from build123d import *

# Parameters (mm, degrees)
BOSS_EXTRUDE7_DEPTH = 15
BOSS_EXTRUDE8_DEPTH = 5
SKETCH3_W           = 4.7625
SKETCH3_H           = 3
SKETCH3_W_2         = 3
SKETCH3_H_2         = 7.9375
CUT_EXTRUDE1_DEPTH  = 15


with BuildPart() as part:
    # Sketch1 → Boss-Extrude7 (new body)
    with BuildSketch(Plane(origin=(0, 0, 0), x_dir=(1, 0, 0), z_dir=(0, 1, 0))):
        Polygon((24.7625, 10.9375), (7.7625, 10.9375), (7.7625, 27.9375), (7.7625, 30.9375), (-3, 30.9375), (-3, 27.9375), (-3, -3), (24.7625, -3), (27.7625, -3), (27.7625, 10.9375), align=None)
        Polygon((0, 0), (4.7625, 0), (24.7625, 0), (24.7625, 7.9375), (4.7625, 7.9375), (4.7625, 27.9375), (0, 27.9375), align=None, mode=Mode.SUBTRACT)
    extrude(amount=BOSS_EXTRUDE7_DEPTH)

    # Sketch2 → Boss-Extrude8 (add)
    with BuildSketch(Plane.XZ):
        Polygon((27.7625, 3), (27.7625, -10.9375), (7.7625, -10.9375), (7.7625, -30.9375), (-3, -30.9375), (-3, 3), align=None)
    extrude(amount=BOSS_EXTRUDE8_DEPTH)

    # Sketch3 → Cut-Extrude1 (cut)
    with BuildSketch(Plane(origin=(0, 15, 0), x_dir=(1, 0, 0), z_dir=(0, 1, 0))):
        with Locations((2.38125, 29.4375)):
            Rectangle(SKETCH3_W, SKETCH3_H)
        with Locations((26.2625, 3.96875)):
            Rectangle(SKETCH3_W_2, SKETCH3_H_2)
    extrude(amount=-CUT_EXTRUDE1_DEPTH, mode=Mode.SUBTRACT)


solid = part.part
The model under review builds one solid part; all positions refer to its coordinate system, in mm. A direction names the side the tool comes from. Round coordinates to 2 decimals unless told otherwise and drop trailing zeros. Write each loop counter-clockwise with the first axis right and the second up, starting at its lowest first coordinate (ties: lowest second). Pieces come first, ordered by that corner, then holes. Notation, with made-up numbers: M 48,32.5 L 104,32.5 A16 cw 104,48.5 Z; hole C 36.25,-13.75 d1. An arc over 180 degrees is marked long. Use a Markdown table: item, result. Add a question column.
Q1. We need section A-A, the plane y = 12. State the section outline as (x, z) points.
Q2. The part is to be moulded in two halves that separate along X. For faces 4 (the face through (4.762, 7, -19)), 5 (the face through (7.762, 5, -21)), 6 (the face through (4, 0, -9)), 7 (the face through (16, 8, -7.938)), say which applies: pulls with the +X half, pulls with the -X half, needs draft (parallel to the pull), parting line crosses it, or undercut.
Q3. We need section C-C, the plane z = -16. State the section outline as (x, y) points.
Q4. Insertion check: pin 1 (4 mm diameter, centred on x = 19, y = 5.5, fed in from -Z); pin 2 (6 mm diameter, centred on y = 9.5, z = -19.5, fed in from +X). Each pin has a flat end and moves straight along its axis. Give the tip position at first contact, or say it passes through.
Q5. We need section D-D, the plane x = 2.5. State the section outline as (y, z) points, plus the area to 3 significant figures.
Q6. Machinability: for faces 1 (the face through (18, 5, -10.938)), 2 (the face through (14, 8, 0)), 3 (the face through (0, 8, -15)), which of the approach directions +Z, -Z, +X, -X, +Y, -Y give a long, thin tool a straight path to every point of the face, cutting with its end or side? Answer none if there is none.
Q7. To check wall thickness, follow line 1 (X direction, y = 9.75, z = -26); line 2 (Z direction, x = 19.5, y = 10); line 3 (Z direction, x = 5.5, y = 10.75). State the ranges of each line that lie inside material, in increasing order.
Q8. We need section B-B, the plane x = 14. State the section outline as (y, z) points, plus the area to 3 significant figures.
Findings below:
| question | item | result |
|---|---|---|
| 1 | outline | M -3,-30.94 L 0,-30.94 L 0,0 L 27.76,0 L 27.76,3 L -3,3 Z; M 4.76,-30.94 L 7.76,-30.94 L 7.76,-10.94 L 27.76,-10.94 L 27.76,-7.94 L 4.76,-7.94 Z |
| 2 | face 4 | undercut |
| 2 | face 5 | pulls with the +X half |
| 2 | face 6 | undercut |
| 2 | face 7 | needs draft |
| 3 | outline | M -3,-5 L 7.76,-5 L 7.76,15 L 4.76,15 L 4.76,0 L 0,0 L 0,15 L -3,15 Z |
| 4 | pin 1 | stops at z = -10.94 |
| 4 | pin 2 | stops at x = 7.76 |
| 5 | outline | M -5,-30.94 L 0,-30.94 L 0,0 L 15,0 L 15,3 L -5,3 Z |
| 5 | area | 215 mm² |
| 6 | face 1 | -Z, +X, +Y, -Y |
| 6 | face 2 | +X, +Y |
| 6 | face 3 | -Z, +Y |
| 7 | line 1 | x = -3 to 0, 4.76 to 7.76 |
| 7 | line 2 | z = -10.94 to -7.94, 0 to 3 |
| 7 | line 3 | z = -30.94 to -7.94, 0 to 3 |
| 8 | outline | M -5,-10.94 L 15,-10.94 L 15,-7.94 L 0,-7.94 L 0,0 L 15,0 L 15,3 L -5,3 Z |
| 8 | area | 160 mm² |
